Build history of the part. All positions in model axes, mm. Face numbers are marked on the shaded views. A direction names the side the tool comes from. Give positions to 0.01 mm unless a question says otherwise; leave off trailing zeros. Order: outer loops, then holes, each group sorted by start corner. A loop starts at its lowest first (then second) coordinate and runs counter-clockwise, first axis right, second up. Notation, with made-up numbers: M 6.5,68 L 17.5,68 A18 ccw 17.5,77 Z; hole C 36,84 d4. An arc over 180 degrees is marked long. Answer as CSV lines item,"result".
from build123d import *

# Parameters (mm, degrees)
F0_W     = 260
F0_H     = 40
F1_DEPTH = 5
F2_W     = 160
F2_H     = 5
F3_DEPTH = 35
F4_W     = 40
F4_H     = 160
F5_DEPTH = 5
F7_DEPTH = 35
F8_R     = 4
F9_DEPTH = 25


with BuildPart() as f1:
    # F0 (on Top) → F1 (new body)
    with BuildSketch(Plane.XY):
        Rectangle(F0_W, F0_H)
    extrude(amount=F1_DEPTH)

    # F2 (on face) → F3 (join)
    with BuildSketch(Plane(origin=(0, 0, 0), x_dir=(1, 0, 0), z_dir=(0, 0, -1))):
        with Locations((-10, 17.5)):
            Rectangle(F2_W, F2_H)
    extrude(amount=F3_DEPTH)

    # F4 (on face) → F5 (join)
    with BuildSketch(Plane(origin=(0, 0, 0), x_dir=(1, 0, 0), z_dir=(0, 0, -1))):
        with Locations((-110, 100)):
            Rectangle(F4_W, F4_H)
    extrude(amount=-F5_DEPTH)

    # F6 (on face) → F7 (join)
    with BuildSketch(Plane(origin=(0, 0, 0), x_dir=(1, 0, 0), z_dir=(0, 0, -1))):
        Polygon((-95, 15), (-90, 15), (-90, 20), (-90, 120), (-95, 120), align=None)
    extrude(amount=F7_DEPTH)

    # F8 (on face) → F9 (cut)
    with BuildSketch(Plane.XY.offset(5)):
        with Locations((-110, -150)):
            Circle(F8_R)
        with Locations((100, 0)):
            Circle(F8_R)
    extrude(amount=-F9_DEPTH, mode=Mode.SUBTRACT)


solid = f1.part
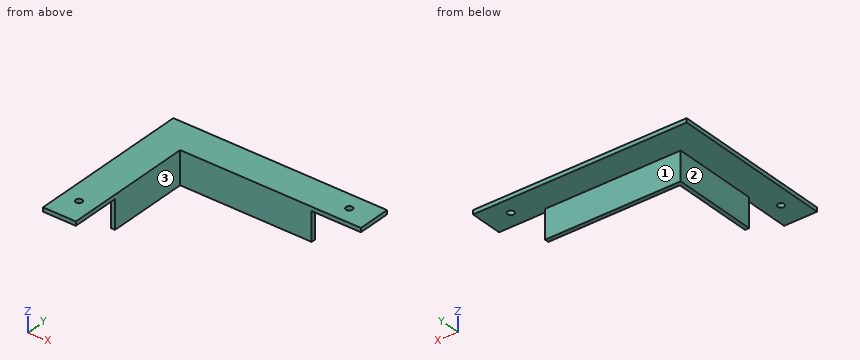
Item 1: Probe line 1 along Y through (x, z) = (100, 1); line 2 along Y through (x, z) = (-110, 3.15); line 3 along Y through (x, z) = (-78, -13.5). List the from-to ranges inside material, lowest first. Write a range as from..to.
Geometry says:
line 1,"y = -20..-4, 4..20"
line 2,"y = -180..-154, -146..20"
line 3,"y = -20..-15"
Item 2: Band-saw the part on B-B (x = -110). Give the cut face in (y, z).
Geometry says:
outline,"M -180,0 L -154,0 L -154,5 L -180,5 Z; M -146,0 L 20,0 L 20,5 L -146,5 Z"
Item 3: Band-saw the part on A-A (y = 0). Give the cut face in (x, z).
Geometry says:
outline,"M -130,0 L 96,0 L 96,5 L -130,5 Z; M 104,0 L 130,0 L 130,5 L 104,5 Z"
Item 4: Band-saw the part on C-C (z = -3). Give the cut face in (x, y).
Geometry says:
outline,"M -95,-120 L -90,-120 L -90,-20 L 70,-20 L 70,-15 L -95,-15 Z"
Item 5: Drop flat-ended pins along their axis: pin 1 (4 mm diameter, centred on x = -92, z = -9, fed in from -Y); pin 2 (3 mm diameter, centred on y = -16.5, z = -7.5, fed in from -X); pin 3 (20 mm diameter, centred on y = -134, z = -6, fed in from +X); pin 4 (10 mm diameter, centred on x = 51.5, y = -26, fed in from +Z). Give the stop position or say it passes through.
Geometry says:
pin 1,"stops at y = -120"
pin 2,"stops at x = -95"
pin 3,"stops at x = -90"
pin 4,"passes through"
Item 6: 3-axis set-ups, long thin cutter, end or side, ignore diameter. For the marked faces 1, 2 and 3: which of +Z, -Z, +X, -X, +Y, -Y reach the whole face in a straight line?
Geometry says:
face 1,"-Z, +X, -X, +Y"
face 2,"-Z, -X, +Y, -Y"
face 3,"+Z, -Z, +X, -Y"
Item 7: Band-saw the part on D-D (x = 63.5). Give the cut face in (y, z).
Geometry says:
outline,"M -20,-35 L -15,-35 L -15,0 L 20,0 L 20,5 L -20,5 Z"
